Verification items for the finished model (mm, model axes). Give positions to 0.01 mm unless a question says otherwise; leave off trailing zeros. Loops run counter-clockwise (first coordinate to the right, second up) from the corner with the lowest first, then second, coordinate; pieces in that order, holes last. Notation, with made-up numbers: (81, 44) - (127, 44) arc R25 cw to (127, 67) - close; hole circle Ø6 at (70.5, -36.75). An arc over 180 degrees is marked (long way). Answer in a Markdown table with one row per item.
Autodesk Inventor part; units mm, degrees
ref_plane "YZ Plane" through (0, 0, 0) normal (1, 0, 0) x (0, 1, 0)
ref_plane "XZ Plane" through (0, 0, 0) normal (0, 1, 0) x (-1, 0, 0)
ref_plane "XY Plane" through (0, 0, 0) normal (0, 0, 1) x (1, 0, 0)
sketch "Sketch1" plane through (0, 0, 0) normal (0, 1, 0) x (-1, 0, 0)
  line L0 (-75, 35) -> (-66, 35) construction
  line L1 (75, 35) -> (75, 26) construction
  line L2 (75, -35) -> (66, -35) construction
  line L3 (-75, -35) -> (-75, -26) construction
  line L4 (-75, 35) -> (75, -35) construction
  line L5 (75, 35) -> (-75, -35) construction
  arc A0 (75, 26) -> (66, 35) centre (66, 26) ccw construction
  arc A1 (66, -35) -> (75, -26) centre (66, -26) ccw
  arc A2 (-75, -26) -> (-66, -35) centre (-66, -26) ccw
  arc A3 (-66, 35) -> (-75, 26) centre (-66, 26) ccw
  line L6 (75, 26) -> (75, 0.5) construction
  line L7 (66, 35) -> (75, 35) construction
  line L8 (-66, 35) -> (66, 35)
  line L9 (-75, 26) -> (-75, 35) construction
  line L10 (-75, -26) -> (-75, 26)
  line L11 (-66, -35) -> (-75, -35) construction
  line L12 (66, -35) -> (-66, -35)
  line L13 (75, -26) -> (75, -35) construction
  circle A4 centre (37.25, 0) radius 8.25
  line L14 (64, 27.375) -> (64, 2.875)
  arc A5 (66.7085, 31.4202) -> (66, 35) centre (66, 33.14) ccw
  arc A6 (64, 2.875) -> (72.3603, 1.0699) centre (68.375, 2.875) ccw
  arc A7 (75, 0.5) -> (72.3603, 1.0699) centre (73.6186, 0.5) ccw
  line L15 (66, 35) -> (66, 35) construction
  line L16 (75, 0.5) -> (75, -26)
  arc A8 (66.7085, 31.4202) -> (64, 27.375) centre (68.375, 27.375) ccw
  point P0 (0, 0)
  point P1 (0, 0)
  dimension "d3" = 70
  dimension "d4" = 150
  dimension "d5" = 16.5
  dimension "d6" = 29.5
  dimension "d7" = 11
  dimension "d10" = 4.375
  dimension "d14" = 36.5
  dimension "d15" = 3.25
  dimension "d17" = 2.375
  dimension "d19" = 9
  dimension "d21" = 2.375
extrude "Extrusion1" add sketch "Sketch1" along normal blind 1
properties part number "Google Pixel - Clear Case Cutout"
Q1. Go/stop test with a flat-tipped pin: P1, Ø2, axis at x = -59, z = 2.5, coming from the -Y side. Record where the tip stops, or that it passes through.
Completed:
| item | result |
|---|---|
| P1 | y = 0 |
Q2. Draft check along X on faces 1 (the face through (-67.533, 0.493, -1.418)), 2 (the face through (1, 1, 0)), 3 (the face through (-64.72, 0.49, 29.78)). Enter one of: +X half, -X half, draft (parallel to the pull), parting line (faces both ways), or undercut.
Completed:
| item | result |
|---|---|
| face 1 | undercut |
| face 2 | draft |
| face 3 | -X half |
Q3. Sectioned sample at B-B (z = -6.5). Record the cut outline in (x, y), and give its area (3 significant figures).
Completed:
| item | result |
|---|---|
| outline | (-75, 0) - (-42.33, 0) - (-42.33, 1) - (-75, 1) - close; (-32.17, 0) - (75, 0) - (75, 1) - (-32.17, 1) - close |
| area | 140 mm^2 |
Q4. Thickness scan on line 1 (Z direction, x = -37.25, y = 0.4); line 2 (X direction, y = 0.9, z = 25.5); line 3 (X direction, y = 0.15, z = 31.5). Record the ranges inside material, lowest first.
Completed:
| item | result |
|---|---|
| line 1 | -35 to -8.25, 8.25 to 35 |
| line 2 | -64 to 75 |
| line 3 | -66.88 to 73.12 |
Q5. Sectioned sample at A-A (x = -37.25). Record the cut outline in (y, z).
Completed:
| item | result |
|---|---|
| outline | (0, -35) - (1, -35) - (1, -8.25) - (0, -8.25) - close; (0, 8.25) - (1, 8.25) - (1, 35) - (0, 35) - close |
Q6. Sectioned sample at D-D (z = 14). Record the cut outline in (x, y).
Completed:
| item | result |
|---|---|
| outline | (-64, 0) - (75, 0) - (75, 1) - (-64, 1) - close |
